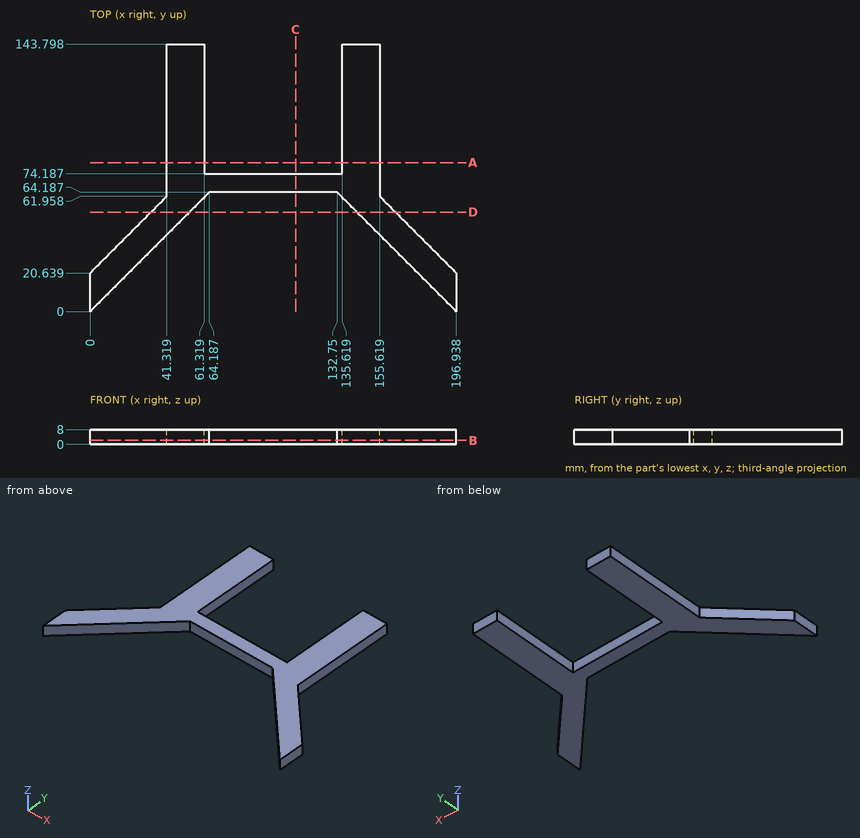
Source: three-view drawing plus pictorial views. Frame: mm from the lowest corner of the part. Give positions to 0.01 mm unless a question says otherwise; leave off trailing zeros. Order: outer loops, then holes, each group sorted by start corner. A loop starts at its lowest first (then second) coordinate and runs counter-clockwise, first axis right, second up. Notation, with made-up numbers: (65.5, 76.5) - (107.5, 76.5) arc R22 cw to (107.5, 113.5) - close; hole circle Ø4 at (22.5, 40.25). An arc over 180 degrees is marked (long way). Put each result on its own line as item: value.
Item 1: Ray query, L1, parallel to X at y = 119.5, z = 1; L2, parallel to Y at x = 76, z = 5.25; L3, parallel to X at y = 27.5, z = 7.75 (1 decimal). Return the intervals inside material, ascending. Write a range as from..to.
Found:
L1: x = 41.32..61.32, 135.62..155.62
L2: y = 64.19..74.19
L3: x = 6.9..27.5, 169.4..190.1
Item 2: Contact query for flat-ended pins moving along their axis: pin 1 (2 mm diameter, centred on x = 81.5, z = 2, fed in from +Y); pin 2 (4 mm diameter, centred on x = 88, z = 2.5, fed in from -Y); pin 3 (1 mm diameter, centred on y = 44, z = 3.5, fed in from +X) (1 decimal). Output: stop coordinate, or through.
Found:
pin 1: stops at y = 74.19
pin 2: stops at y = 64.19
pin 3: stops at x = 174.1
Item 3: Section query D-D, the plane y = 53.5. Return loops of the section in (x, z), then the cut area to 3 significant figures.
Found:
outline: (32.86, 0) - (53.5, 0) - (53.5, 8) - (32.86, 8) - close; (143.44, 0) - (164.08, 0) - (164.08, 8) - (143.44, 8) - close
area: 330 mm^2
Item 4: Section query A-A, the plane y = 80. Return loops of the section in (x, z), then the cut area to 3 significant figures.
Found:
outline: (41.32, 0) - (61.32, 0) - (61.32, 8) - (41.32, 8) - close; (135.62, 0) - (155.62, 0) - (155.62, 8) - (135.62, 8) - close
area: 320 mm^2
Item 5: Section query C-C, the plane x = 110.5. Return loops of the section in (y, z), then the cut area to 3 significant figures.
Found:
outline: (64.19, 0) - (74.19, 0) - (74.19, 8) - (64.19, 8) - close
area: 80.0 mm^2
Item 6: Section query B-B, the plane z = 2.25. Return loops of the section in (x, y), then the cut area to 3 significant figures.
Found:
outline: (0, 0) - (64.19, 64.19) - (132.75, 64.19) - (196.94, 0) - (196.94, 20.64) - (155.62, 61.96) - (155.62, 143.8) - (135.62, 143.8) - (135.62, 74.19) - (61.32, 74.19) - (61.32, 143.8) - (41.32, 143.8) - (41.32, 61.96) - (0, 20.64) - close
area: 6,160 mm^2
